Read the model definition and answer for the solid it produces. Units are mm, in the model's axes. Give positions to 0.01 mm unless a question says otherwise; leave off trailing zeros. Write each loop counter-clockwise with the first axis right and the second up, starting at its lowest first coordinate (ties: lowest second). Pieces come first, ordered by that corner, then holes. Notation, with made-up numbers: (64.5, -5) - (78.5, -5) arc R13 cw to (78.5, 10) - close; hole circle Ø1 at (-25.5, -31.5). An arc over 180 degrees is marked (long way). Answer as CSV lines item,"result".
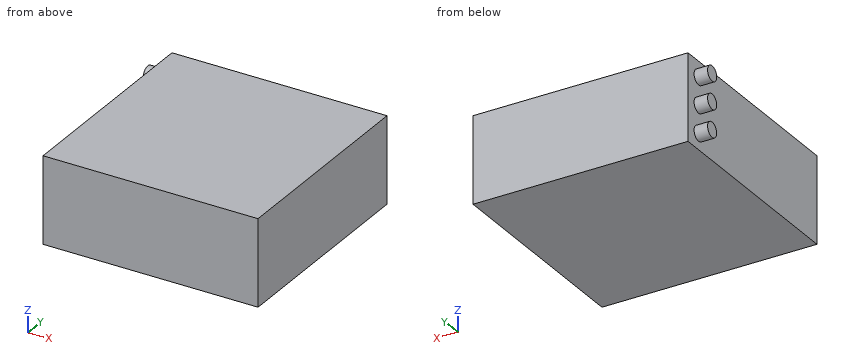
```python
from build123d import *

# Parameters (mm, degrees)
SKETCH1_W           = 430
SKETCH1_H           = 426
BOSS_EXTRUDE1_DEPTH = 173
SKETCH2_R           = 15
BOSS_EXTRUDE2_DEPTH = 27


with BuildPart() as part:
    # Sketch1 → Boss-Extrude1 (new body)
    with BuildSketch(Plane.XY):
        with Locations((215, 213)):
            Rectangle(SKETCH1_W, SKETCH1_H)
    extrude(amount=BOSS_EXTRUDE1_DEPTH)

    # Sketch2 → Boss-Extrude2 (add)
    with BuildSketch(Plane.ZY):
        with Locations(Location((86.5, 391, 0), (0, 0, 180))):
            Circle(SKETCH2_R)
        with Locations(Location((31.5, 391, 0), (0, 0, 180))):
            Circle(SKETCH2_R)
        with Locations(Location((141.5, 391, 0), (0, 0, 180))):
            Circle(SKETCH2_R)
    extrude(amount=BOSS_EXTRUDE2_DEPTH)


solid = part.part
```
(1) A cutting plane is placed at D-D (y = 78). Write down the section's boundary in (x, z), and give its area (3 significant figures).
Worked out:
outline,"(0, 0) - (430, 0) - (430, 173) - (0, 173) - close"
area,"74,400 mm^2"
(2) A cutting plane is placed at A-A (z = 132.5). Write down the section's boundary in (x, y), and give its area (3 significant figures).
Worked out:
outline,"(-27, 379) - (0, 379) - (0, 0) - (430, 0) - (430, 426) - (0, 426) - (0, 403) - (-27, 403) - close"
area,"184,000 mm^2"
(3) This flat-tipped pin is pushed along its axis until it touches: P1, Ø1.5, axis at y = 147, z = 84.5, coming from the -X side. Where does it stop, or does it pass through?
Worked out:
P1,"stops at x = 0"
(4) Find the intervals of material crossed by L1, parallel to X at y = 220, z = 110.5, in increasing order.
Worked out:
L1,"x = 0 to 430"
(5) A cutting plane is placed at C-C (z = 31.5). Write down the section's boundary in (x, y).
Worked out:
outline,"(-27, 376) - (0, 376) - (0, 0) - (430, 0) - (430, 426) - (0, 426) - (0, 406) - (-27, 406) - close"
(6) A cutting plane is placed at B-B (y = 391). Write down the section's boundary in (x, z).
Worked out:
outline,"(-27, 16.5) - (0, 16.5) - (0, 0) - (430, 0) - (430, 173) - (0, 173) - (0, 156.5) - (-27, 156.5) - (-27, 126.5) - (0, 126.5) - (0, 101.5) - (-27, 101.5) - (-27, 71.5) - (0, 71.5) - (0, 46.5) - (-27, 46.5) - close"
